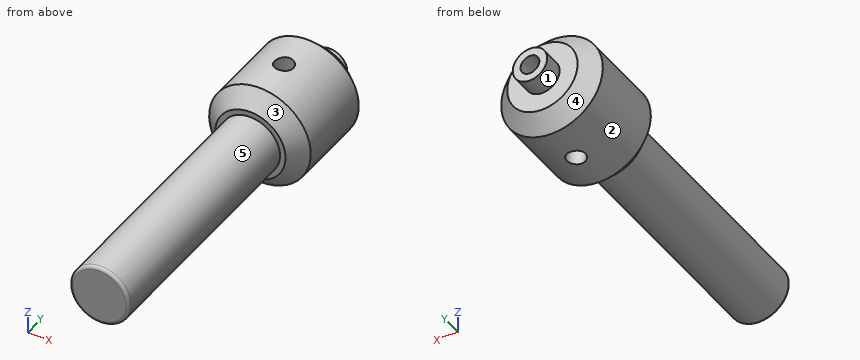
```python
from build123d import *

# Parameters (mm, degrees)
CHAMFER1_SIZE           = 10
FILLET1_R               = 2
HOLE1_D                 = 12
HOLE1_DEPTH             = 23
CUT_EXTRUDE1_DEPTH      = 245.361412666
CUT_EXTRUDE1_DEPTH_BACK = 245.361412666
SKETCH4_R               = 6


with BuildPart() as part:
    # Sketch1 → Revolve1 (revolve)
    with BuildSketch(Plane.XY, mode=Mode.PRIVATE) as revolve1_sk:
        Polygon((0, 0), (0, 240), (11, 240), (11, 227), (32.5, 227), (32.5, 157), (19, 157), (19, 0), align=None)
    revolve(revolve1_sk.sketch.rotate(Axis((0, 0, 0), (0, 1, 0)), 90), axis=Axis((0, 0, 0), (0, 1, 0)))

    # Chamfer1
    chamfer1_edges = [part.edges().sort_by_distance(p)[0] for p in [
        (0, 157, 32.5),
        (0, 227, 32.5),
    ]]
    chamfer(chamfer1_edges, length=CHAMFER1_SIZE)

    # Fillet1
    fillet1_edges = [part.edges().sort_by_distance(p)[0] for p in [
        (0, 0, 19),
    ]]
    fillet(fillet1_edges, radius=FILLET1_R)

    # Hole1
    with Locations(Plane(origin=(0, 240, 0), x_dir=(1, 0, 0), z_dir=(0, 1, 0))):
        with Locations((0, 0)):
            Hole(HOLE1_D / 2, depth=HOLE1_DEPTH)

    # Sketch4 → Cut-Extrude1 (cut, two sides: drawn at the far end of the back side and taken through both)
    with BuildSketch(Plane.XY.offset(-CUT_EXTRUDE1_DEPTH_BACK)):
        with Locations((0, 192)):
            Circle(SKETCH4_R)
    extrude(amount=CUT_EXTRUDE1_DEPTH + CUT_EXTRUDE1_DEPTH_BACK, mode=Mode.SUBTRACT)


solid = part.part
```
Verification items for the finished model (mm, model axes). Face numbers are marked on the shaded views. A direction names the side the tool comes from. Round coordinates to 2 decimals unless told otherwise and drop trailing zeros. Order: outer loops, then holes, each group sorted by start corner. A loop starts at its lowest first (then second) coordinate and runs counter-clockwise, first axis right, second up. Notation, with made-up numbers: (73.25, 65.25) - (131.25, 65.25) arc R10 cw to (131.25, 76.25) - close; hole circle Ø10 at (65.25, -2.5). An arc over 180 degrees is marked (long way). Use CSV: the item, a comma, the result in double quotes.
(1) Section check A-A on x = 0. Record the boundary of the cut face in (y, z), and give its area (3 significant figures).
Entries:
outline,"(0, -17) arc R2 ccw to (2, -19) - (157, -19) - (157, -22.5) - (167, -32.5) - (186, -32.5) - (186, 32.5) - (167, 32.5) - (157, 22.5) - (157, 19) - (2, 19) arc R2 ccw to (0, 17) - close; (198, -32.5) - (217, -32.5) - (227, -22.5) - (227, -11) - (240, -11) - (240, -6) - (217, -6) - (217, 6) - (240, 6) - (240, 11) - (227, 11) - (227, 22.5) - (217, 32.5) - (198, 32.5) - close"
area,"9,540 mm^2"
(2) Thickness scan on probe 1 along Y at (x, z) = (0, 12.5); probe 2 along X at (y, z) = (192, 10); probe 3 along X at (y, z) = (190.5, 26). Record the ranges inside material, lowest first. Write a range as from..to.
Entries:
probe 1,"0..186, 198..227"
probe 2,"-30.92..-6, 6..30.92"
probe 3,"-19.5..-5.81, 5.81..19.5"
(3) Gauge pin test, flat ends, axial feed: pin 1 Ø6 at (x, z) = (-19, -21.5) entering from -Y; pin 2 Ø3 at (x, z) = (1, -15) entering from +Y; pin 3 Ø3 at (x, y) = (8, 46.5) entering from -Z. Record the tip position at first contact, or that the pin passes through.
Entries:
pin 1,"y = 160.19"
pin 2,"y = 227"
pin 3,"z = -17.85"
(4) Section check C-C on y = 48. Record the boundary of the cut face in (x, z).
Entries:
outline,"circle Ø38 at (0, 0)"
(5) Section check D-D on y = 192. Record the boundary of the cut face in (x, z), and give its area (3 significant figures).
Entries:
outline,"(-6, -31.94) - (-6, 31.94) arc R32.5 ccw to start; (6, -31.94) arc R32.5 ccw to (6, 31.94) - close"
area,"2,540 mm^2"
(6) Section check B-B on z = 0. Record the boundary of the cut face in (x, y).
Entries:
outline,"(-32.5, 167) - (-22.5, 157) - (-19, 157) - (-19, 2) arc R2 ccw to (-17, 0) - (17, 0) arc R2 ccw to (19, 2) - (19, 157) - (22.5, 157) - (32.5, 167) - (32.5, 217) - (22.5, 227) - (11, 227) - (11, 240) - (6, 240) - (6, 217) - (-6, 217) - (-6, 240) - (-11, 240) - (-11, 227) - (-22.5, 227) - (-32.5, 217) - close; hole circle Ø12 at (0, 192)"
(7) Access from +Z, -Z, +X, -X, +Y, -Y to the whole of each face (thin tool, end or side, straight path). Record for the marked faces 1 and 2.
Entries:
face 1,"+Y"
face 2,"+Y, -Y"
(8) Mould release check, pull along Y, two halves, no side actions. Record for the marked faces 3, 4 and 5: released by +Y, released by -Y, zero draft, split by the parting line, or undercut.
Entries:
face 3,"released by -Y"
face 4,"released by +Y"
face 5,"zero draft"
